```python
from build123d import *

# Parameters (mm, degrees)
SKETCH1_R           = 4
BOSS_EXTRUDE1_DEPTH = 10
SKETCH2_R           = 4.8
BOSS_EXTRUDE2_DEPTH = 2.3
CHAMFER1_SIZE       = 0.8
CHAMFER2_SIZE       = 0.5
SKETCH3_R           = 2.55
CUT_EXTRUDE1_DEPTH  = 3
SKETCH4_R           = 3.25
CUT_EXTRUDE2_DEPTH  = 10
CUT_EXTRUDE3_DEPTH  = 5


with BuildPart() as part:
    # Sketch1 → Boss-Extrude1 (new body)
    with BuildSketch(Plane.XY):
        Circle(SKETCH1_R)
    extrude(amount=BOSS_EXTRUDE1_DEPTH)

    # Sketch2 → Boss-Extrude2 (add)
    with BuildSketch(Plane.XY.offset(10)):
        Circle(SKETCH2_R)
    extrude(amount=BOSS_EXTRUDE2_DEPTH)

    # Chamfer1
    chamfer1_edges = [part.edges().sort_by_distance(p)[0] for p in [
        (-4.8, 0, 12.3),
    ]]
    chamfer(chamfer1_edges, length=CHAMFER1_SIZE)

    # Chamfer2
    chamfer2_edges = [part.edges().sort_by_distance(p)[0] for p in [
        (-4, 0, 0),
    ]]
    chamfer(chamfer2_edges, length=CHAMFER2_SIZE)

    # Sketch3 → Cut-Extrude1 (cut)
    with BuildSketch(Plane.XY.offset(12.3)):
        Circle(SKETCH3_R)
    extrude(amount=-CUT_EXTRUDE1_DEPTH, mode=Mode.SUBTRACT)

    # Sketch4 → Cut-Extrude2 (cut)
    with BuildSketch(Plane(origin=(0, 0, 0), x_dir=(-1, 0, 0), z_dir=(0, 0, -1))):
        Circle(SKETCH4_R)
    extrude(amount=-CUT_EXTRUDE2_DEPTH, mode=Mode.SUBTRACT)

    # Sketch5 → Cut-Extrude3 (cut, symmetric)
    with BuildSketch(Plane(origin=(0, 0, 0), x_dir=(1, 0, 0), z_dir=(0, 1, 0))):
        Polygon((-3, -10), (-2.375, -10), (-2.375, -3.5), (-1.125, -3.5), (-1.125, -10), (1.125, -10), (1.125, -3.5), (2.375, -3.5), (2.375, -10), (3, -10), (3, -3), (0.625, -3), (0.625, -9.25), (-0.625, -9.25), (-0.625, -3), (-3, -3), align=None)
    extrude(amount=CUT_EXTRUDE3_DEPTH, both=True, mode=Mode.SUBTRACT)


solid = part.part
```
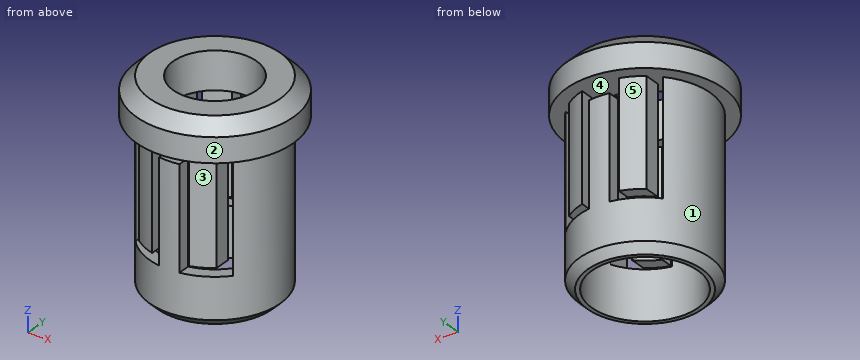
The listing builds one solid part. Answer for the finished solid, in the listing's coordinates (mm). Face numbers are marked on the shaded views. A direction names the side the tool comes from. Coordinates: 2 decimals unless noted, no trailing zeros. Write each loop counter-clockwise with the first axis right and the second up, starting at its lowest first coordinate (ties: lowest second). Pieces come first, ordered by that corner, then holes. Notation, with made-up numbers: (-37, 9.5) - (18, 9.5) arc R28 cw to (18, 40.5) - close; hole circle Ø11 at (-26.5, 11). An arc over 180 degrees is marked (long way). Return JSON: item names as keys, results as strings. Group by question number.
1. Determine the mould class of the marked faces 3, 4 and 5 for opening direction X: released by +X, released by -X, zero draft, split by the parting line, or undercut.
2. A cutting plane is placed at A-A, the plane z = 4. Give the number of separate pieces and of enclosed holes in the cut face, plus the area to 3 significant figures.
3. A cutting plane is placed at D-D, the plane z = 10.25. Determine the outline of the cut face in (x, y), plus the area to 3 significant figures.
4. Which of the six approach directions +Z, -Z, +X, -X, +Y, -Y give full straight-line access (tool end or side, diameter ignored) to the marked faces 1 and 2?
5. Given pin 1 (3 mm diameter, centred on x = 2.5, z = 5.5, fed in from +Y); pin 2 (0.8 mm diameter, centred on y = -2.5, z = 6, fed in from -X); pin 3 (1.1 mm diameter, centred on y = 3, z = 7, fed in from -X), each flat-ended and moving along its own axis, determine where each tip first touches the part or whether it passes through.
6. Straight lines are drawn through the part: L1, parallel to Y at x = 0, z = 11.4; L2, parallel to Y at x = 0, z = 2.5; L3, parallel to Z at x = 1.75, y = -2.5. For each, find the intervals that lie inside material, in ascending order.
7. A cutting plane is placed at C-C, the plane x = 0. Determine the outline of the cut face in (y, z), plus the area to 3 significant figures.
8. A cutting plane is placed at B-B, the plane y = 0. Determine the outline of the cut face in (x, z), plus the area to 3 significant figures.
Ans:
{
 "1": {"face 3": "released by +X", "face 4": "undercut", "face 5": "released by -X"},
 "2": {"separate pieces": "8", "enclosed holes": "0", "area": "12.6 mm²"},
 "3": {"outline": "circle Ø9.6 at (0, 0); hole circle Ø5.1 at (0, 0)", "area": "52.0 mm²"},
 "4": {"face 1": "-Z", "face 2": "+Z, -Z"},
 "5": {"pin 1": "y = 3.84", "pin 2": "x = -3.4", "pin 3": "x = -3.16"},
 "6": {"L1": "-4.8 to -2.55, 2.55 to 4.8", "L2": "-4 to -3.25, 3.25 to 4", "L3": "10 to 12.3"},
 "7": {"outline": "(-4.8, 10) - (-2.55, 10) - (-2.55, 12.3) - (-4, 12.3) - (-4.8, 11.5) - close; (-4, 0.5) - (-3.5, 0) - (-3.25, 0) - (-3.25, 9.25) - (-4, 9.25) - close; (2.55, 10) - (4.8, 10) - (4.8, 11.5) - (4, 12.3) - (2.55, 12.3) - close; (3.25, 0) - (3.5, 0) - (4, 0.5) - (4, 9.25) - (3.25, 9.25) - close", "area": "23.3 mm²"},
 "8": {"outline": "(-4.8, 10) - (-4, 10) - (-4, 0.5) - (-3.5, 0) - (-3.25, 0) - (-3.25, 10) - (-2.55, 10) - (-2.55, 12.3) - (-4, 12.3) - (-4.8, 11.5) - close; (2.55, 10) - (3.25, 10) - (3.25, 0) - (3.5, 0) - (4, 0.5) - (4, 10) - (4.8, 10) - (4.8, 11.5) - (4, 12.3) - (2.55, 12.3) - close", "area": "24.5 mm²"}
}
